Read the model definition and answer for the solid it produces. Units are mm, in the model's axes. Face numbers are marked on the shaded views. A direction names the side the tool comes from. Coordinates: 2 decimals unless noted, no trailing zeros. Write each loop counter-clockwise with the first axis right and the second up, starting at its lowest first coordinate (ties: lowest second). Pieces come first, ordered by that corner, then holes. Notation, with made-up numbers: (-22.5, 54) -> (-0.5, 54) arc R17 cw to (-0.5, 84) -> close; hole circle Ø3 at (79.5, -0.75). An arc over 180 degrees is marked (long way). One line per item, written item: value. Start each with the question number.
1. For a pull along Y with two mould halves and no side action, classify the marked faces 1, 2, 3 and 4 as pulls with the +Y half, pulls with the -Y half, needs draft (parallel to the pull), parting line crosses it, or undercut.
2. Find section D-D, the plane x = -22. Write down the section's boundary in (y, z), and give its area (3 significant figures).
3. Find section A-A, the plane x = 0. Write down the section's boundary in (y, z), and give its area (3 significant figures).
4. Given P1, Ø1.5, axis at x = 1, z = 7.5, coming from the +Y side; P2, Ø5, axis at x = 17.5, z = 9.5, coming from the +Y side; P3, Ø4, axis at y = -24.5, z = 5.5, coming from the -X side, each flat-ended and moving along its own axis, determine where each tip first touches the part or whether it passes through.
5. Find section B-B, the plane y = 2. Write down the section's boundary in (x, z), and give its area (3 significant figures).
6. Consider line 1 along Y through (x, z) = (0, 4.5); line 2 along Y through (x, z) = (0, 11.25); line 3 along X through (y, z) = (-25, 1.5). Determine where each line is inside the solid, lowest interval first.
7. Find section C-C, the plane z = 2.5. Write down the section's boundary in (x, y).
8. For the marked faces 5, 6 and 7, determine the directions among +Z, -Z, +X, -X, +Y, -Y from which every point of the face is accessible in a straight line to the end or side of a thin tool.
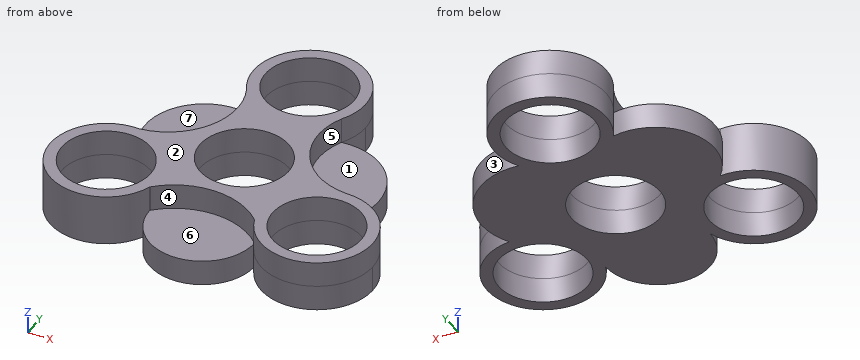
```python
from build123d import *

# Parameters (mm, degrees)
F0_R       = 13.97
F0_R_2     = 11.049
F1_DEPTH   = 6.35
F2_R       = 11.049
F3_DEPTH   = 6.35
F4_DEPTH   = 6.35
F1_FACE_R  = 11.049
F1_FACE1_R = 11.049
F5_DEPTH   = 6.35
F6_DEPTH   = 25.4


with BuildPart() as f1:
    # F0 (on Top) → F1 (new body)
    with BuildSketch(Plane.XY):
        with BuildLine():
            ThreePointArc((11.8822308851, 23.133334825), (0, 16.51), (-11.8822308851, 23.133334825))
            ThreePointArc((-11.8822308851, 23.133334825), (-12.4666938835, 7.4417065656), (-25.5122345043, -1.2980110694))
            ThreePointArc((-25.5122345043, -1.2980110694), (-16.2103497858, -5.6794469472), (-12.4264543073, -15.24))
            ThreePointArc((-12.4264543073, -15.24), (-12.6043267068, -17.4621872669), (-13.1334144003, -19.627786734))
            ThreePointArc((-13.1334144003, -19.627786734), (0.0089857965, -14.1771556489), (13.141390917, -19.6518243979))
            ThreePointArc((13.141390917, -19.6518243979), (15.0105571103, -7.1454187867), (26.2086928391, -1.2712618454))
            ThreePointArc((26.2086928391, -1.2712618454), (12.551407877, 7.1187703581), (11.8822308851, 23.133334825))
        make_face()
        Circle(F0_R, mode=Mode.SUBTRACT)
        Circle(F0_R)
        Circle(F0_R_2, mode=Mode.SUBTRACT)
        with BuildLine():
            ThreePointArc((11.8822308851, 23.133334825), (13.4379251647, 26.6612217572), (13.97, 30.48))
            ThreePointArc((13.97, 30.48), (-3.8187782428, 43.9179251647), (-11.8822308851, 23.133334825))
            ThreePointArc((-11.8822308851, 23.133334825), (0, 16.51), (11.8822308851, 23.133334825))
        make_face()
        with Locations((0, 30.48)):
            Circle(F0_R_2, mode=Mode.SUBTRACT)
        with BuildLine():
            ThreePointArc((-12.4264543073, -15.24), (-16.2103497858, -5.6794469472), (-25.5122345043, -1.2980110694))
            ThreePointArc((-25.5122345043, -1.2980110694), (-37.9736477628, -23.0585351374), (-13.1334144003, -19.627786734))
            ThreePointArc((-13.1334144003, -19.627786734), (-12.6043267068, -17.4621872669), (-12.4264543073, -15.24))
        make_face()
        with Locations((-26.3964543073, -15.24)):
            Circle(F0_R_2, mode=Mode.SUBTRACT)
        with BuildLine():
            ThreePointArc((27.3639044924, -1.3035391817), (26.786025252, -1.2971860413), (26.2086928391, -1.2712618454))
            ThreePointArc((26.2086928391, -1.2712618454), (15.0105571103, -7.1454187867), (13.141390917, -19.6518243979))
            ThreePointArc((13.141390917, -19.6518243979), (28.6311427014, -29.0301076059), (40.3664543073, -15.24))
            ThreePointArc((40.3664543073, -15.24), (36.6110560883, -5.7098997667), (27.3639044924, -1.3035391817))
        make_face()
        with Locations((26.3964543073, -15.24)):
            Circle(F0_R_2, mode=Mode.SUBTRACT)
        with Locations((26.3964543073, -15.24)):
            Circle(F0_R_2)
        Circle(F0_R_2)
        with Locations((0, 30.48)):
            Circle(F0_R_2)
        with Locations((-26.3964543073, -15.24)):
            Circle(F0_R_2)
        with BuildLine():
            ThreePointArc((27.3639044924, -1.3035391817), (26.7866325748, -1.275449849), (26.2086928391, -1.2712618454))
            ThreePointArc((26.2086928391, -1.2712618454), (26.786025252, -1.2971860413), (27.3639044924, -1.3035391817))
        make_face()
    extrude(amount=F1_DEPTH)

    # F2 (on face) → F3 (cut)
    with BuildSketch(Plane.XY.offset(6.35)):
        with Locations((-26.3964543073, -15.24)):
            Circle(F2_R)
        with Locations((0, 30.48)):
            Circle(F2_R)
        with Locations((26.3964543073, -15.24)):
            Circle(F2_R)
    extrude(amount=-F3_DEPTH, mode=Mode.SUBTRACT)

    # F2 (on face) → F4 (cut)
    with BuildSketch(Plane.XY.offset(6.35)):
        Circle(F2_R)
    extrude(amount=-F4_DEPTH, mode=Mode.SUBTRACT)

    # F0 (on Top) + F1_face (on face) + F1_face1 (on face) → F5 (join)
    with BuildSketch(Plane.XY):
        with BuildLine():
            ThreePointArc((11.8822308851, 23.133334825), (0, 16.51), (-11.8822308851, 23.133334825))
            ThreePointArc((-11.8822308851, 23.133334825), (-12.4666938835, 7.4417065656), (-25.5122345043, -1.2980110694))
            ThreePointArc((-25.5122345043, -1.2980110694), (-16.2103497858, -5.6794469472), (-12.4264543073, -15.24))
            ThreePointArc((-12.4264543073, -15.24), (-12.6043267068, -17.4621872669), (-13.1334144003, -19.627786734))
            ThreePointArc((-13.1334144003, -19.627786734), (0.0089857965, -14.1771556489), (13.141390917, -19.6518243979))
            ThreePointArc((13.141390917, -19.6518243979), (15.0105571103, -7.1454187867), (26.2086928391, -1.2712618454))
            ThreePointArc((26.2086928391, -1.2712618454), (12.551407877, 7.1187703581), (11.8822308851, 23.133334825))
        make_face()
        Circle(F0_R, mode=Mode.SUBTRACT)
        with BuildLine():
            ThreePointArc((11.8822308851, 23.133334825), (13.4379251647, 26.6612217572), (13.97, 30.48))
            ThreePointArc((13.97, 30.48), (-3.8187782428, 43.9179251647), (-11.8822308851, 23.133334825))
            ThreePointArc((-11.8822308851, 23.133334825), (0, 16.51), (11.8822308851, 23.133334825))
        make_face()
        with Locations((0, 30.48)):
            Circle(F0_R_2, mode=Mode.SUBTRACT)
        Circle(F0_R)
        Circle(F0_R_2, mode=Mode.SUBTRACT)
        with BuildLine():
            ThreePointArc((-12.4264543073, -15.24), (-16.2103497858, -5.6794469472), (-25.5122345043, -1.2980110694))
            ThreePointArc((-25.5122345043, -1.2980110694), (-37.9736477628, -23.0585351374), (-13.1334144003, -19.627786734))
            ThreePointArc((-13.1334144003, -19.627786734), (-12.6043267068, -17.4621872669), (-12.4264543073, -15.24))
        make_face()
        with Locations((-26.3964543073, -15.24)):
            Circle(F0_R_2, mode=Mode.SUBTRACT)
        with BuildLine():
            ThreePointArc((27.3639044924, -1.3035391817), (26.786025252, -1.2971860413), (26.2086928391, -1.2712618454))
            ThreePointArc((26.2086928391, -1.2712618454), (15.0105571103, -7.1454187867), (13.141390917, -19.6518243979))
            ThreePointArc((13.141390917, -19.6518243979), (28.6311427014, -29.0301076059), (40.3664543073, -15.24))
            ThreePointArc((40.3664543073, -15.24), (36.6110560883, -5.7098997667), (27.3639044924, -1.3035391817))
        make_face()
        with Locations((26.3964543073, -15.24)):
            Circle(F0_R_2, mode=Mode.SUBTRACT)
        with Locations((26.3964543073, -15.24)):
            Circle(F0_R_2)
        with Locations((0, 30.48)):
            Circle(F0_R_2)
        with Locations((-26.3964543073, -15.24)):
            Circle(F0_R_2)
        Circle(F0_R_2)
        with BuildLine():
            ThreePointArc((13.141390917, -19.6518243979), (0.0089857965, -14.1771556489), (-13.1334144003, -19.627786734))
            ThreePointArc((-13.1334144003, -19.627786734), (-0.0079653205, -32.7058821649), (13.141390917, -19.6518243979))
        make_face()
        with BuildLine():
            ThreePointArc((27.3639044924, -1.3035391817), (27.2624668136, 15.7547428761), (11.8822308851, 23.133334825))
            ThreePointArc((11.8822308851, 23.133334825), (12.551407877, 7.1187703581), (26.2086928391, -1.2712618454))
            ThreePointArc((26.2086928391, -1.2712618454), (26.7866325748, -1.275449849), (27.3639044924, -1.3035391817))
        make_face()
        with BuildLine():
            ThreePointArc((-25.5122345043, -1.2980110694), (-12.4666938835, 7.4417065656), (-11.8822308851, 23.133334825))
            ThreePointArc((-11.8822308851, 23.133334825), (-27.5570644864, 15.8604734571), (-25.5122345043, -1.2980110694))
        make_face()
        with BuildLine():
            ThreePointArc((27.3639044924, -1.3035391817), (26.7866325748, -1.275449849), (26.2086928391, -1.2712618454))
            ThreePointArc((26.2086928391, -1.2712618454), (26.786025252, -1.2971860413), (27.3639044924, -1.3035391817))
        make_face()
    with BuildSketch(Plane(origin=(-0.004664817, 0.0791445283, 6.35), x_dir=(1, 0, 0), z_dir=(0, 0, 1))):
        with BuildLine():
            ThreePointArc((13.146055734, -19.7309689261), (37.7870163213, -23.4137257416), (26.213357656, -1.3504063737))
            ThreePointArc((26.213357656, -1.3504063737), (12.556072694, 7.0396258298), (11.886895702, 23.0541902967))
            ThreePointArc((11.886895702, 23.0541902967), (0.004664817, 44.3708554717), (-11.8775660681, 23.0541902967))
            ThreePointArc((-11.8775660681, 23.0541902967), (-12.4620290666, 7.3625620373), (-25.5075696873, -1.3771555977))
            ThreePointArc((-25.5075696873, -1.3771555977), (-37.9689829458, -23.1376796657), (-13.1287495833, -19.7069312623))
            ThreePointArc((-13.1287495833, -19.7069312623), (0.0136506135, -14.2563001772), (13.146055734, -19.7309689261))
        make_face()
        with Locations((-26.3917894904, -15.3191445283)):
            Circle(F1_FACE_R, mode=Mode.SUBTRACT)
        with Locations((26.4011191243, -15.3191445283)):
            Circle(F1_FACE_R, mode=Mode.SUBTRACT)
        with Locations((0.004664817, -0.0791445283)):
            Circle(F1_FACE_R, mode=Mode.SUBTRACT)
        with Locations((0.004664817, 30.4008554717)):
            Circle(F1_FACE_R, mode=Mode.SUBTRACT)
    with BuildSketch(Plane(origin=(-0.0103051715, 0.1748402862, 0), x_dir=(1, 0, 0), z_dir=(0, 0, -1))):
        with BuildLine():
            ThreePointArc((26.2189980105, 1.4461021316), (37.7926566758, 23.5094214995), (13.1516960884, 19.8266646841))
            ThreePointArc((13.1516960884, 19.8266646841), (0.019290968, 14.3519959351), (-13.1231092288, 19.8026270202))
            ThreePointArc((-13.1231092288, 19.8026270202), (-37.9633425914, 23.2333754236), (-25.5019293328, 1.4728513557))
            ThreePointArc((-25.5019293328, 1.4728513557), (-12.4563887121, -7.2668662794), (-11.8719257136, -22.9584945388))
            ThreePointArc((-11.8719257136, -22.9584945388), (0.0103051715, -44.2751597138), (11.8925360565, -22.9584945388))
            ThreePointArc((11.8925360565, -22.9584945388), (12.5617130485, -6.9439300719), (26.2189980105, 1.4461021316))
        make_face()
        with Locations((-26.3861491359, 15.4148402862)):
            Circle(F1_FACE1_R, mode=Mode.SUBTRACT)
        with Locations((26.4067594788, 15.4148402862)):
            Circle(F1_FACE1_R, mode=Mode.SUBTRACT)
        with Locations((0.0103051715, 0.1748402862)):
            Circle(F1_FACE1_R, mode=Mode.SUBTRACT)
        with Locations((0.0103051715, -30.3051597138)):
            Circle(F1_FACE1_R, mode=Mode.SUBTRACT)
    extrude(amount=F5_DEPTH, dir=(0, 0, 1))

    # F2 (on face) → F6 (cut)
    with BuildSketch(Plane.XY.offset(6.35)):
        with Locations((-26.3964543073, -15.24)):
            Circle(F2_R)
        Circle(F2_R)
        with Locations((0, 30.48)):
            Circle(F2_R)
        with Locations((26.3964543073, -15.24)):
            Circle(F2_R)
    extrude(amount=-F6_DEPTH, mode=Mode.SUBTRACT)


solid = f1.part
```
Answer block:
1. face 1: undercut
1. face 2: needs draft
1. face 3: undercut
1. face 4: pulls with the -Y half
2. outline: (-28.5, 0) -> (-25.38, 0) -> (-25.38, 12.7) -> (-28.5, 12.7) -> close; (-5.1, 0) -> (21.47, 0) -> (21.47, 6.35) -> (-0.5, 6.35) -> (-0.5, 12.7) -> (-5.1, 12.7) -> close
2. area: 238 mm2
3. outline: (-32.71, 0) -> (-11.05, 0) -> (-11.05, 12.7) -> (-14.18, 12.7) -> (-14.18, 6.35) -> (-32.71, 6.35) -> close; (11.05, 0) -> (19.43, 0) -> (19.43, 12.7) -> (11.05, 12.7) -> close; (41.53, 0) -> (44.45, 0) -> (44.45, 12.7) -> (41.53, 12.7) -> close
3. area: 301 mm2
4. P1: stops at y = 44.45
4. P2: stops at y = 3.9
4. P3: stops at x = -38.33
5. outline: (-27.81, 0) -> (-10.87, 0) -> (-10.87, 12.7) -> (-17.24, 12.7) -> (-17.24, 6.35) -> (-27.81, 6.35) -> close; (10.87, 0) -> (28.92, 0) -> (28.92, 6.35) -> (17.17, 6.35) -> (17.17, 12.7) -> (10.87, 12.7) -> close
5. area: 303 mm2
6. line 1: y = -32.71 to -11.05, 11.05 to 19.43, 41.53 to 44.45
6. line 2: y = -14.18 to -11.05, 11.05 to 19.43, 41.53 to 44.45
6. line 3: x = -36.39 to -31.58, -21.22 to -16.4, -11.96 to 11.97, 16.4 to 21.22, 31.58 to 36.39
7. outline: (-25.51, -1.3) arc R13.97 ccw (long way) to (-13.13, -19.63) arc R13.14 ccw to (13.14, -19.65) arc R13.97 ccw (long way) to (27.36, -1.3) arc R16.09 ccw to (11.88, 23.13) arc R13.97 ccw (long way) to (-11.88, 23.13) arc R14.72 ccw to start; hole circle Ø22.1 at (-26.4, -15.24); hole circle Ø22.1 at (0, 0); hole circle Ø22.1 at (0, 30.48); hole circle Ø22.1 at (26.4, -15.24)
8. face 5: +Z, +X
8. face 6: +Z, -Y
8. face 7: +Z, -X
